from build123d import *

# Parameters (mm, degrees)
SKETCH1_R           = 25.4
BOSS_EXTRUDE1_DEPTH = 6.35
SKETCH2_R           = 15.875
BOSS_EXTRUDE2_DEPTH = 9.525
SKETCH3_R           = 4.7625
CUT_EXTRUDE1_DEPTH  = 15.875


with BuildPart() as part:
    # Sketch1 → Boss-Extrude1 (new body)
    with BuildSketch(Plane.XY):
        Circle(SKETCH1_R)
    extrude(amount=BOSS_EXTRUDE1_DEPTH)

    # Sketch2 → Boss-Extrude2 (add)
    with BuildSketch(Plane.XY.offset(6.35)):
        with Locations(Location((0, 0, 0), (0, 0, 180))):
            Circle(SKETCH2_R)
    extrude(amount=BOSS_EXTRUDE2_DEPTH)

    # Sketch3 → Cut-Extrude1 (cut)
    with BuildSketch(Plane.XY.offset(15.875)):
        Circle(SKETCH3_R)
    extrude(amount=-CUT_EXTRUDE1_DEPTH, mode=Mode.SUBTRACT)


solid = part.part
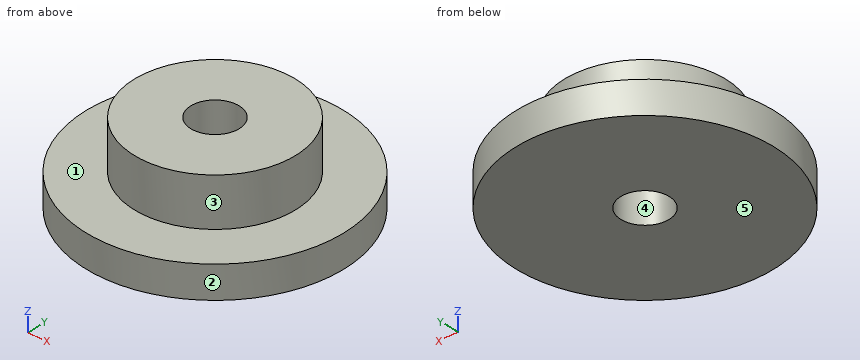
Part model, mm, in its own coordinate system. Face numbers are marked on the shaded views. A direction names the side the tool comes from. Coordinates: 2 decimals unless noted, no trailing zeros. Order: outer loops, then holes, each group sorted by start corner. A loop starts at its lowest first (then second) coordinate and runs counter-clockwise, first axis right, second up. Notation, with made-up numbers: M 46.5,85 L 54.5,85 A22 cw 54.5,114 Z; hole C -11,80.25 d6. An arc over 180 degrees is marked long. Use a Markdown table: item, result.
(1) Tool access for the marked faces 1 and 2: list every direction of +Z, -Z, +X, -X, +Y, -Y with a clear straight run to the whole face (end or side of a thin tool).
A:
| item | result |
|---|---|
| face 1 | +Z |
| face 2 | +Z, -Z |
(2) Flat gauge pins, fed straight in: pin 1 (1.5 mm diameter, centred on y = -18.5, z = 4, fed in from +X); pin 2 (5.5 mm diameter, centred on x = 0, y = 0, fed in from -Z); pin 3 (5 mm diameter, centred on y = 9, z = 5, fed in from -X); pin 4 (6 mm diameter, centred on y = -13, z = 12.5, fed in from +X). Where does each tip first touch, or does it go through?
A:
| item | result |
|---|---|
| pin 1 | stops at x = 18.17 |
| pin 2 | passes through |
| pin 3 | stops at x = -24.55 |
| pin 4 | stops at x = 12.33 |
(3) Cut at C-C on z = 3. Write the cut outline in (x, y) (1 decimal), then the cut area to 3 significant figures.
A:
| item | result |
|---|---|
| outline | C 0,0 d50.8; hole C 0,0 d9.5 |
| area | 1,960 mm^2 |
(4) Pull direction X, two halves, no side cores. Call the marked faces 3, 4 and 5: released by +X, released by -X, zero draft, split by the parting line, or undercut.
A:
| item | result |
|---|---|
| face 3 | split by the parting line |
| face 4 | undercut |
| face 5 | zero draft |
(5) Cut at D-D on x = -10. Write the cut outline in (y, z) (3 decimals).
A:
| item | result |
|---|---|
| outline | M -23.349,0 L 23.349,0 L 23.349,6.35 L 12.329,6.35 L 12.329,15.875 L -12.329,15.875 L -12.329,6.35 L -23.349,6.35 Z |
(6) Probe L1, parallel to Y at x = 0, z = 6.5 (1 decimal); L2, parallel to Y at x = 0, z = 5; L3, parallel to Z at x = 22.5, y = -2.5. List the from-to ranges inside material, lowest first.
A:
| item | result |
|---|---|
| L1 | y = -15.9 to -4.8, 4.8 to 15.9 |
| L2 | y = -25.4 to -4.76, 4.76 to 25.4 |
| L3 | z = 0 to 6.35 |
